Check sheet for the drawn part. Datum: minimum x, y, z corner. Units: mm. Give positions to 0.01 mm unless a question says otherwise; leave off trailing zeros. Write each loop counter-clockwise with the first axis right and the second up, starting at its lowest first coordinate (ties: lowest second). Pieces come first, ordered by that corner, then holes. Notation, with made-up numbers: (68.5, -1.5) -> (74.5, -1.5) arc R31 cw to (74.5, 28.5) -> close; hole circle Ø3 at (48, 59). An arc over 180 degrees is marked (long way). Write item = value, one per line. Start each with the question number.
1. Depth check by flat-ended pin: P1, Ø4.5, axis at x = 10, y = 30, coming from the -Z side; P2, Ø1, axis at x = 3.5, z = 3, coming from the +Y side. Enter the tip coordinate at first touch or a pass-through.
2. Cross-section at D-D, the plane y = 3. Record the cut outline in (x, z).
3. Cross-section at C-C, the plane z = 2.95. Record the cut outline in (x, y), plus the area to 3 significant figures.
4. Mould release check, pull along Y, two halves, no side actions. Record for the marked faces 1, 2, 3 and 4: pulls with the +Y half, pulls with the -Y half, needs draft (parallel to the pull), parting line crosses it, or undercut.
5. Thickness scan on line 1 along Y through (x, z) = (10, 3.3); line 2 along X through (y, z) = (3, 1.05); line 3 along Y through (x, z) = (15.5, 2.5). Record the ranges inside material, lowest first.
6. Cross-section at A-A, the plane y = 10. Record the cut outline in (x, z), plus the area to 3 significant figures.
7. Cross-section at B-B, the plane x = 10. Record the cut outline in (y, z), plus the area to 3 significant figures.
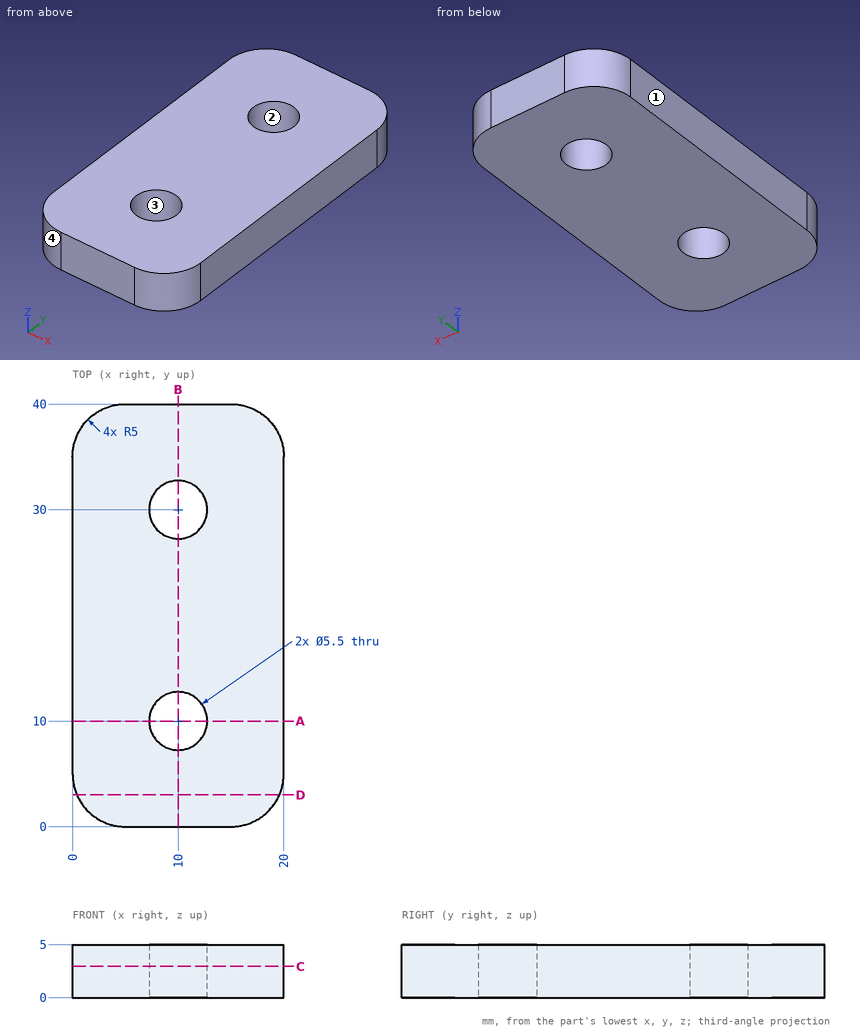
Answers:
q1.P1 = through
q1.P2 = 39.9
q2.outline = (0.42, 0) -> (19.58, 0) -> (19.58, 5) -> (0.42, 5) -> close
q3.outline = (0, 5) arc R5 ccw to (5, 0) -> (15, 0) arc R5 ccw to (20, 5) -> (20, 35) arc R5 ccw to (15, 40) -> (5, 40) arc R5 ccw to (0, 35) -> close; hole circle Ø5.5 at (10, 10); hole circle Ø5.5 at (10, 30)
q3.area = 731 mm^2
q4.face_1 = needs draft
q4.face_2 = undercut
q4.face_3 = undercut
q4.face_4 = pulls with the -Y half
q5.line_1 = 0 to 7.25, 12.75 to 27.25, 32.75 to 40
q5.line_2 = 0.42 to 19.58
q5.line_3 = 0.03 to 39.97
q6.outline = (0, 0) -> (7.25, 0) -> (7.25, 5) -> (0, 5) -> close; (12.75, 0) -> (20, 0) -> (20, 5) -> (12.75, 5) -> close
q6.area = 72.5 mm^2
q7.outline = (0, 0) -> (7.25, 0) -> (7.25, 5) -> (0, 5) -> close; (12.75, 0) -> (27.25, 0) -> (27.25, 5) -> (12.75, 5) -> close; (32.75, 0) -> (40, 0) -> (40, 5) -> (32.75, 5) -> close
q7.area = 145 mm^2
